Part model, mm, in its own coordinate system. Give positions to 0.01 mm unless a question says otherwise; leave off trailing zeros. Order: outer loops, then holes, each group sorted by start corner. A loop starts at its lowest first (then second) coordinate and runs counter-clockwise, first axis right, second up. Notation, with made-up numbers: M -18,7.5 L 37,7.5 A17 ccw 37,17.5 Z; hole C 56.5,80.25 d8. An arc over 180 degrees is marked long. Answer as a JSON object with one key per item and string values.
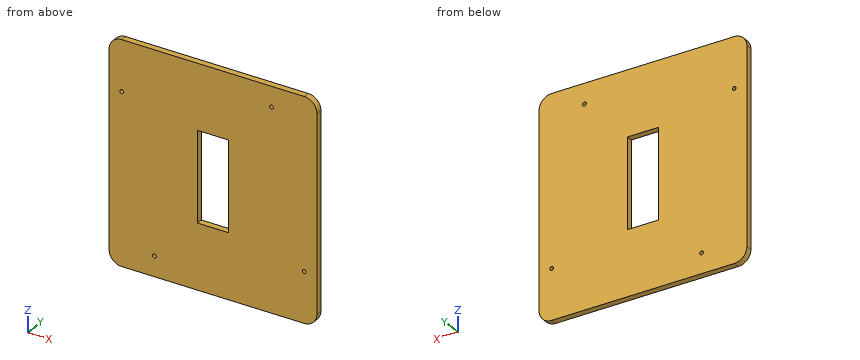
from build123d import *

# Parameters (mm, degrees)
RESSALTO_EXTRUS_O1_DEPTH = 5
ESBO_O2_R                = 1.5
CORTE_EXTRUS_O1_DEPTH    = 5
ESBO_O3_W                = 25
ESBO_O3_H                = 71.5
CORTE_EXTRUS_O2_DEPTH    = 5


with BuildPart() as part:
    # Esboço1 → Ressalto-extrusão1 (new body)
    with BuildSketch(Plane(origin=(0, 0, 0), x_dir=(1, 0, 0), z_dir=(0, 1, 0))):
        with BuildLine():
            Line((-25.463589741, 142.264378701), (119.536410259, 142.264378701))
            ThreePointArc((119.536410259, 142.264378701), (126.607478071, 139.335446513), (129.536410259, 132.264378701))
            Line((129.536410259, 132.264378701), (129.536410259, -22.735621299))
            ThreePointArc((129.536410259, -22.735621299), (126.607478071, -29.806689111), (119.536410259, -32.735621299))
            Line((119.536410259, -32.735621299), (-25.463589741, -32.735621299))
            ThreePointArc((-25.463589741, -32.735621299), (-32.534657553, -29.806689111), (-35.463589741, -22.735621299))
            Line((-35.463589741, -22.735621299), (-35.463589741, 132.264378701))
            ThreePointArc((-35.463589741, 132.264378701), (-32.534657553, 139.335446513), (-25.463589741, 142.264378701))
        make_face()
    extrude(amount=RESSALTO_EXTRUS_O1_DEPTH)

    # Esboço2 → Corte-extrusão1 (cut)
    with BuildSketch(Plane(origin=(0, 5, 0), x_dir=(1, 0, 0), z_dir=(0, 1, 0))):
        with Locations(Location((-25.463589741, 7.264378701, 0), (0, 0, 270))):
            Circle(ESBO_O2_R)
        with Locations(Location((0.536410259, 126.264378701, 0), (0, 0, 270))):
            Circle(ESBO_O2_R)
        with Locations(Location((119.536410259, 102.264378701, 0), (0, 0, 270))):
            Circle(ESBO_O2_R)
        with Locations(Location((93.536410259, -16.735621299, 0), (0, 0, 270))):
            Circle(ESBO_O2_R)
    extrude(amount=-CORTE_EXTRUS_O1_DEPTH, mode=Mode.SUBTRACT)

    # Esboço3 → Corte-extrusão2 (cut)
    with BuildSketch(Plane(origin=(0, 5, 0), x_dir=(1, 0, 0), z_dir=(0, 1, 0))):
        with Locations((47.036410259, 54.764378701)):
            Rectangle(ESBO_O3_W, ESBO_O3_H)
    extrude(amount=-CORTE_EXTRUS_O2_DEPTH, mode=Mode.SUBTRACT)


solid = part.part
1. Probe line 1 along X through (y, z) = (3.55, -28); line 2 along X through (y, z) = (0.8, -7.5); line 3 along Z through (x, y) = (53, 2.8). List the from-to ranges inside material, lowest first.
Worked answers:
{"line 1": "x = -35.46 to 34.54, 59.54 to 129.54", "line 2": "x = -35.46 to -26.94, -23.98 to 129.54", "line 3": "z = -142.26 to -90.51, -19.01 to 32.74"}
2. Cut at C-C on y = 3.15. Give the cut face in (x, z), plus the area to 3 significant figures.
Worked answers:
{"outline": "M -35.46,-132.26 A10 ccw -25.46,-142.26 L 119.54,-142.26 A10 ccw 129.54,-132.26 L 129.54,22.74 A10 ccw 119.54,32.74 L -25.46,32.74 A10 ccw -35.46,22.74 Z; hole C -25.46,-7.26 d3; hole C 0.54,-126.26 d3; hole M 34.54,-90.51 L 59.54,-90.51 L 59.54,-19.01 L 34.54,-19.01 Z; hole C 93.54,16.74 d3; hole C 119.54,-102.26 d3", "area": "27,000 mm^2"}
3. Pin check, flat tip, straight feed: P1, Ø2.5, axis at x = 93.54, z = 16.74, coming from the +Y side. Stop position of the tip, or through.
Worked answers:
{"P1": "passes through"}
4. Cut at A-A on x = 44. Give the cut face in (y, z), plus the area to 4 significant figures.
Worked answers:
{"outline": "M 0,-142.26 L 5,-142.26 L 5,-90.51 L 0,-90.51 Z; M 0,-19.01 L 5,-19.01 L 5,32.74 L 0,32.74 Z", "area": "517.5 mm^2"}
5. Cut at B-B on z = -84.5. Give the cut face in (x, y), plus the area to 3 significant figures.
Worked answers:
{"outline": "M -35.46,0 L 34.54,0 L 34.54,5 L -35.46,5 Z; M 59.54,0 L 129.54,0 L 129.54,5 L 59.54,5 Z", "area": "700 mm^2"}
